```python
from build123d import *

# Parameters (mm, degrees)
SKETCH1_W           = 114.3
SKETCH1_H           = 254
BOSS_EXTRUDE1_DEPTH = 1.5875
SKETCH2_W           = 3.175
SKETCH2_H           = 50.8
BOSS_EXTRUDE2_DEPTH = 50.8
CUT_EXTRUDE1_DEPTH  = 50
SKETCH4_R           = 3.96875
CUT_EXTRUDE2_DEPTH  = 50
SKETCH5_R           = 3.96875
CUT_EXTRUDE3_DEPTH  = 100
CHAMFER1_SIZE       = 15
FILLET1_R           = 15


with BuildPart() as part:
    # Sketch1 → Boss-Extrude1 (new, symmetric)
    with BuildSketch(Plane(origin=(0, 0, 0), x_dir=(1, 0, 0), z_dir=(0, 1, 0))):
        Rectangle(SKETCH1_W, SKETCH1_H)
    extrude(amount=BOSS_EXTRUDE1_DEPTH, both=True)

    # Sketch2 → Boss-Extrude2 (add)
    with BuildSketch(Plane(origin=(0, 1.5875, 0), x_dir=(1, 0, 0), z_dir=(0, 1, 0))):
        with Locations((46.0375, -50.8)):
            Rectangle(SKETCH2_W, SKETCH2_H)
        with Locations((-46.0375, -50.8)):
            Rectangle(SKETCH2_W, SKETCH2_H)
    extrude(amount=BOSS_EXTRUDE2_DEPTH)

    # Sketch3 → Cut-Extrude1 (cut, symmetric)
    with BuildSketch(Plane(origin=(0, 0, 0), x_dir=(0, 0, -1), z_dir=(1, 0, 0))):
        Polygon((-25.4, 1.5875), (-25.4, 52.3875), (-30.4, 52.3875), align=None)
        Polygon((-76.2, 52.3875), (-71.2, 52.3875), (-76.2, 1.5875), align=None)
    extrude(amount=CUT_EXTRUDE1_DEPTH, both=True, mode=Mode.SUBTRACT)

    # Sketch4 → Cut-Extrude2 (cut, symmetric)
    with BuildSketch(Plane(origin=(0, 0, 0), x_dir=(0, 0, -1), z_dir=(1, 0, 0))):
        with Locations((-50.8, 26.9875)):
            Circle(SKETCH4_R)
    extrude(amount=CUT_EXTRUDE2_DEPTH, both=True, mode=Mode.SUBTRACT)

    # Sketch5 → Cut-Extrude3 (cut)
    with BuildSketch(Plane(origin=(0, 1.5875, 0), x_dir=(1, 0, 0), z_dir=(0, 1, 0))):
        with Locations(Location((31.75, -101.6, 0), (0, 0, 270))):
            Circle(SKETCH5_R)
        with Locations(Location((-31.75, -101.6, 0), (0, 0, 270))):
            Circle(SKETCH5_R)
        with Locations(Location((31.75, 101.6, 0), (0, 0, 270))):
            Circle(SKETCH5_R)
        with Locations(Location((-31.75, 101.6, 0), (0, 0, 270))):
            Circle(SKETCH5_R)
        with Locations(Location((0, 0, 0), (0, 0, 270))):
            Circle(SKETCH5_R)
        with BuildLine():
            Line((-1.984375, -101.6), (-1.984375, -71.6))
            ThreePointArc((-1.984375, -71.6), (0, -69.615625), (1.984375, -71.6))
            Line((1.984375, -71.6), (1.984375, -101.6))
            ThreePointArc((1.984375, -101.6), (0, -103.584375), (-1.984375, -101.6))
        make_face()
        with BuildLine():
            Line((-1.984375, -46.2), (-1.984375, -16.2))
            ThreePointArc((-1.984375, -16.2), (0, -14.215625), (1.984375, -16.2))
            Line((1.984375, -16.2), (1.984375, -46.2))
            ThreePointArc((1.984375, -46.2), (0, -48.184375), (-1.984375, -46.2))
        make_face()
        with BuildLine():
            Line((-1.984375, 16.2), (-1.984375, 46.2))
            ThreePointArc((-1.984375, 46.2), (0, 48.184375), (1.984375, 46.2))
            Line((1.984375, 46.2), (1.984375, 16.2))
            ThreePointArc((1.984375, 16.2), (0, 14.215625), (-1.984375, 16.2))
        make_face()
        with BuildLine():
            Line((-1.984375, 71.6), (-1.984375, 101.6))
            ThreePointArc((-1.984375, 101.6), (0, 103.584375), (1.984375, 101.6))
            Line((1.984375, 101.6), (1.984375, 71.6))
            ThreePointArc((1.984375, 71.6), (0, 69.615625), (-1.984375, 71.6))
        make_face()
        with BuildLine():
            Line((33.734375, -46.2), (33.734375, -71.6))
            ThreePointArc((33.734375, -71.6), (31.75, -73.584375), (29.765625, -71.6))
            Line((29.765625, -71.6), (29.765625, -46.2))
            ThreePointArc((29.765625, -46.2), (31.75, -44.215625), (33.734375, -46.2))
        make_face()
        with BuildLine():
            Line((33.734375, 16.2), (33.734375, -16.2))
            ThreePointArc((33.734375, -16.2), (31.75, -18.184375), (29.765625, -16.2))
            Line((29.765625, -16.2), (29.765625, 16.2))
            ThreePointArc((29.765625, 16.2), (31.75, 18.184375), (33.734375, 16.2))
        make_face()
        with BuildLine():
            Line((33.734375, 71.6), (33.734375, 46.2))
            ThreePointArc((33.734375, 46.2), (31.75, 44.215625), (29.765625, 46.2))
            Line((29.765625, 46.2), (29.765625, 71.6))
            ThreePointArc((29.765625, 71.6), (31.75, 73.584375), (33.734375, 71.6))
        make_face()
        with BuildLine():
            Line((-29.765625, -46.2), (-29.765625, -71.6))
            ThreePointArc((-29.765625, -71.6), (-31.75, -73.584375), (-33.734375, -71.6))
            Line((-33.734375, -71.6), (-33.734375, -46.2))
            ThreePointArc((-33.734375, -46.2), (-31.75, -44.215625), (-29.765625, -46.2))
        make_face()
        with BuildLine():
            Line((-29.765625, 16.2), (-29.765625, -16.2))
            ThreePointArc((-29.765625, -16.2), (-31.75, -18.184375), (-33.734375, -16.2))
            Line((-33.734375, -16.2), (-33.734375, 16.2))
            ThreePointArc((-33.734375, 16.2), (-31.75, 18.184375), (-29.765625, 16.2))
        make_face()
        with BuildLine():
            Line((-29.765625, 71.6), (-29.765625, 46.2))
            ThreePointArc((-29.765625, 46.2), (-31.75, 44.215625), (-33.734375, 46.2))
            Line((-33.734375, 46.2), (-33.734375, 71.6))
            ThreePointArc((-33.734375, 71.6), (-31.75, 73.584375), (-29.765625, 71.6))
        make_face()
        Polygon((57.15, 38), (57.15, 23), (47.15, 27.550166045), (47.15, 34.812409498), align=None)
        Polygon((-47.15, 27.550166045), (-57.15, 23), (-57.15, 38), (-47.15, 34.812409498), align=None)
        Polygon((47.15, -101.550166045), (57.15, -97), (57.15, -112), (47.15, -108.812409498), align=None)
        Polygon((-57.15, -112), (-57.15, -97), (-47.15, -101.550166045), (-47.15, -108.812409498), align=None)
    extrude(amount=-CUT_EXTRUDE3_DEPTH, mode=Mode.SUBTRACT)

    # Chamfer1
    chamfer1_edges = [part.edges().sort_by_distance(p)[0] for p in [
        (-57.15, 0, -127),
        (57.15, 0, -127),
    ]]
    chamfer(chamfer1_edges, length=CHAMFER1_SIZE)

    # Fillet1
    fillet1_edges = [part.edges().sort_by_distance(p)[0] for p in [
        (-46.0375, 52.3875, 71.2),
        (-46.0375, 52.3875, 30.4),
        (46.0375, 52.3875, 30.4),
        (46.0375, 52.3875, 71.2),
    ]]
    fillet(fillet1_edges, radius=FILLET1_R)


solid = part.part
```
Geometry check sheet. Reference: the model listing, model coordinates, mm. A direction names the side the tool comes from. Coordinates: 2 decimals unless noted, no trailing zeros. Order: outer loops, then holes, each group sorted by start corner. A loop starts at its lowest first (then second) coordinate and runs counter-clockwise, first axis right, second up. Notation, with made-up numbers: (-12, 85.5) - (24, 85.5) arc R23 ccw to (24, 110.5) - close; hole circle Ø9 at (87.5, 8). An arc over 180 degrees is marked (long way). Use one line per item in the form item = value.
1. Gauge pin test, flat ends, axial feed: pin 1 (1.6 mm diameter, centred on y = -0.5, z = -31.5, fed in from +X); pin 2 (12 mm diameter, centred on y = 17.5, z = 18.5, fed in from -X); pin 3 (12.5 mm diameter, centred on x = 31.75, z = 101.6, fed in from +Y); pin 4 (9 mm diameter, centred on y = 26.99, z = 50.8, fed in from -X) (3 decimals). Record the tip position at first contact, or that the pin passes through.
Here are the results:
pin_1 = 47.15
pin_2 = through
pin_3 = 1.59
pin_4 = -47.625
2. Section check C-C (y = 43.5). Record the boundary of the cut face in (x, z) (3 decimals).
Here are the results:
outline = (-47.625, 30.298) - (-44.45, 30.298) - (-44.45, 71.302) - (-47.625, 71.302) - close; (44.45, 30.298) - (47.625, 30.298) - (47.625, 71.302) - (44.45, 71.302) - close
3. Section check A-A (z = 50.8). State how many separate pieces and enclosed holes the cut face has, then the cut area to 3 significant figures.
Here are the results:
separate_pieces = 5
enclosed_holes = 0
area = 610 mm²
4. Section check B-B (z = 83). Record the boundary of the cut face in (x, y), then the cut area to 3 significant figures.
Here are the results:
outline = (-57.15, -1.59) - (-1.98, -1.59) - (-1.98, 1.59) - (-57.15, 1.59) - close; (1.98, -1.59) - (57.15, -1.59) - (57.15, 1.59) - (1.98, 1.59) - close
area = 350 mm²
5. Scan lines: line 1 (X direction, y = 0.35, z = 0); line 2 (X direction, y = -0.9, z = -101.6); line 3 (X direction, y = 24.5, z = 55) (3 decimals). Record each from-to range of solid material in increasing order.
Here are the results:
line_1 = -57.15 to -33.73, -29.77 to -3.97, 3.97 to 29.77, 33.73 to 57.15
line_2 = -57.15 to -35.72, -27.78 to -1.98, 1.98 to 27.78, 35.72 to 57.15
line_3 = -47.625 to -44.45, 44.45 to 47.625
6. Section check D-D (x = -23). Record the boundary of the cut face in (y, z), then the cut area to 3 significant figures.
Here are the results:
outline = (-1.59, -127) - (1.59, -127) - (1.59, 127) - (-1.59, 127) - close
area = 806 mm²
7. Access from +Z, -Z, +X, -X, +Y, -Y to the whole of each face (thin tool, end or side, straight path). Record for faces 1 (the face through (-47.625, 21, 51)), 2 (the face through (47.625, 21, 51)), 3 (the face through (44.45, 21, 51)), 4 (the face through (52.1, 0, 99.3)).
Here are the results:
face_1 = +Z, -Z, -X, +Y
face_2 = +Z, -Z, +X, +Y
face_3 = +Z, -Z, +Y
face_4 = +X, +Y, -Y
8. Draft check along Z on faces 5 (the face through (46.02, 48.4, 67.79)), 6 (the face through (-46.06, 48.4, 33.81)), 7 (the face through (27.876, 0.022, -102.46)). Enter one of: pulls with the +Z half, pulls with the -Z half, needs draft (parallel to the pull), parting line crosses it, or undercut.
Here are the results:
face_5 = pulls with the +Z half
face_6 = pulls with the -Z half
face_7 = undercut
